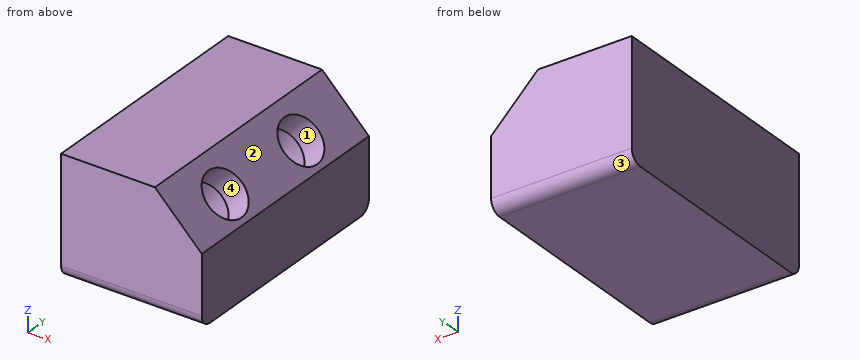
from build123d import *

# Parameters (mm, degrees)
F0_W     = 60
F0_H     = 100
F1_DEPTH = 50
F2_SIZE  = 20
F4_D     = 20
F4_DEPTH = 12
F4_TIP   = 6.0086061903
F6_R     = 5
F7_R     = 5


with BuildPart() as f1:
    # F0 (on Top) → F1 (new body)
    with BuildSketch(Plane.XY):
        with Locations((30, 50)):
            Rectangle(F0_W, F0_H)
    extrude(amount=F1_DEPTH)

    # F2
    f2_edges = [f1.edges().sort_by_distance(p)[0] for p in [
        (60, 50, 50),
    ]]
    chamfer(f2_edges, length=F2_SIZE)

    # F4
    with Locations(Plane(origin=(45, 0, 45), x_dir=(0.7071067812, 0, -0.7071067812), z_dir=(0.7071067812, 0, 0.7071067812))):
        with Locations((8.8761840016, 26.199977845), (8.8761840016, 71.5014504518)):
            Hole(F4_D / 2, depth=F4_DEPTH)
            with Locations((0, 0, -(F4_DEPTH + F4_TIP / 2))):  # 118° drill point
                Cone(0, F4_D / 2, F4_TIP, mode=Mode.SUBTRACT)

    # F6
    f6_edges = [f1.edges().sort_by_distance(p)[0] for p in [
        (30, 0, 0),
    ]]
    fillet(f6_edges, radius=F6_R)

    # F7
    f7_edges = [f1.edges().sort_by_distance(p)[0] for p in [
        (30, 100, 0),
    ]]
    fillet(f7_edges, radius=F7_R)


solid = f1.part
For this review, take the finished solid that the model builds, in its own axes (mm). Face numbers are marked on the shaded views. Round coordinates to 2 decimals unless told otherwise and drop trailing zeros. Order: outer loops, then holes, each group sorted by start corner. A loop starts at its lowest first (then second) coordinate and runs counter-clockwise, first axis right, second up. Notation, with made-up numbers: M 47,-21.75 L 74,-21.75 A20 cw 74,-16.75 Z; hole C 57.5,-30 d9. An arc over 180 degrees is marked long. Write each question's results on one line, items separated by ' | '. Start each with the question number.
1. Add section A-A (y = 55). State the section outline as (x, z) points.
2. To check wall thickness, follow L1, parallel to Y at x = 49, z = 28.5; L2, parallel to Y at x = 46, z = 29; L3, parallel to Z at x = 54, y = 31. State the ranges of each line that lie inside material, in increasing order. Write a range as [from, to].
3. Add section B-B (z = 31.5). State how many separate pieces and enclosed holes the cut face has, then the cut area to 3 significant figures.
4. Draft analysis for pull direction Z (two halves, no side actions). For the marked faces 1, 2, 3 and 4, state which applies: pulls with the +Z half, pulls with the -Z half, needs draft (parallel to the pull), parting line crosses it, or undercut.
Output values:
1) outline: M 0,0 L 60,0 L 60,30 L 40,50 L 0,50 Z
2) L1: [0, 17.93], [34.47, 63.23], [79.77, 100] | L2: [0, 16.71], [35.69, 62.01], [80.99, 100] | L3: [0, 29.04]
3) separate pieces: 1 | enclosed holes: 2 | area: 5,190 mm^2
4) face 1: undercut | face 2: pulls with the +Z half | face 3: pulls with the -Z half | face 4: undercut
